Input: part model. Units: mm. Frame: model coordinates. A direction names the side the tool comes from. Give positions to 0.01 mm unless a question says otherwise; leave off trailing zeros. Order: outer loops, then holes, each group sorted by start corner. A loop starts at its lowest first (then second) coordinate and runs counter-clockwise, first axis right, second up. Notation, with made-up numbers: (70, -30.75) - (110, -30.75) arc R23 cw to (110, 1.25) - close; hole circle Ø7 at (85.5, 74). An arc over 180 degrees is marked (long way). Answer in a Markdown table with one row per item. Add a question column.
1. Ray query, line 1 (Y direction, x = -13, z = -17); line 2 (X direction, y = 4.25, z = -113); line 3 (Z direction, x = -24, y = 4.5). Return the intervals inside material, ascending. Write a range as [from, to].
2. Contact query for flat-ended pins moving along their axis: pin 1 (10 mm diameter, centred on x = 4.5, y = 7.5, fed in from -Z); pin 2 (3.5 mm diameter, centred on y = 3, z = -133.5, fed in from +X); pin 3 (13.5 mm diameter, centred on x = -2, z = -101.5, fed in from +Y); pin 4 (2 mm diameter, centred on x = -6, y = 4.5, fed in from +Z). Output: stop coordinate, or through.
3. Section query B-B on y = 15. Return loops of the section in (x, z).
4. Section query A-A on z = -97.5. Return loops of the section in (x, y).
5. Access query for faces 1 (the face through (-7.412, 12.409, -194.498)), 2 (the face through (-23.074, 0.285, 5.322)). Directions: +Z, -Z, +X, -X, +Y, -Y. A direction counts if a zero-diameter tool reaches every point of the face in a straight line with its end or side. Return the directions, or none.
```python
from build123d import *

# Parameters (mm, degrees)
SKETCH1_W           = 15
SKETCH1_H           = 200
SKETCH1_W_2         = 47.5
SKETCH1_H_2         = 10
BOSS_EXTRUDE1_DEPTH = 5
SKETCH4_R           = 2
BOSS_EXTRUDE3_DEPTH = 15
FILLET5_R           = 1
FILLET6_R           = 1


with BuildPart() as part:
    # Sketch1 → Boss-Extrude1 (new body)
    with BuildSketch(Plane(origin=(0, 0, 0), x_dir=(1, 0, 0), z_dir=(0, 1, 0))):
        Polygon((-31.25, -10), (16.25, -10), (0, 0), (-15, 0), align=None)
        with Locations((-7.5, 100)):
            Rectangle(SKETCH1_W, SKETCH1_H)
        with Locations((-7.5, -15)):
            Rectangle(SKETCH1_W_2, SKETCH1_H_2)
    extrude(amount=BOSS_EXTRUDE1_DEPTH)

    # Sketch4 → Boss-Extrude3 (add)
    with BuildSketch(Plane(origin=(0, 5, 0), x_dir=(1, 0, 0), z_dir=(0, 1, 0))):
        with Locations(Location((-7.5, 192.5, 0), (0, 0, 270))):
            Circle(SKETCH4_R)
    extrude(amount=BOSS_EXTRUDE3_DEPTH)

    # Fillet5
    fillet5_edges = [part.edges().sort_by_distance(p)[0] for p in [
        (-31.25, 5, 15),
        (-7.5, 0, -200),
        (0, 0, -100),
        (8.125, 0, 5),
        (16.25, 0, 15),
        (-7.5, 0, 20),
        (-31.25, 0, 15),
        (-23.125, 0, 5),
        (-7.5, 5, 20),
        (-15, 2.5, 0),
        (-15, 2.5, -200),
        (0, 2.5, -200),
        (0, 2.5, 0),
        (16.25, 2.5, 10),
        (-31.25, 2.5, 10),
        (16.25, 5, 15),
        (8.125, 5, 5),
        (-7.5, 5, -194.5),
        (-7.5, 20, -194.5),
        (0, 5, -100),
        (-7.5, 5, -200),
        (-15, 5, -100),
        (-23.125, 5, 5),
        (-15, 0, -100),
    ]]
    fillet(fillet5_edges, radius=FILLET5_R)

    # Fillet6
    # the kernel refuses this fillet: 1 mm, written as the material it takes off along each edge
    with BuildSketch(Plane(origin=(15.25, 4, 19), x_dir=(1, 0, 0), z_dir=(0, 0, 1))) as fillet6_piece_1_section:
        Polygon((0, 0), (FILLET6_R, 0), (FILLET6_R, FILLET6_R), (0, FILLET6_R), align=None)
    fillet6_piece_1 = extrude(amount=FILLET6_R, mode=Mode.PRIVATE)
    fillet6_piece_1 = fillet6_piece_1 - Plane(origin=(15.25, 4, 19), x_dir=(-0.7071067811865475, -0.7071067811865475, 0), z_dir=(0, 0, 1)) * Sphere(FILLET6_R, mode=Mode.PRIVATE)
    add(fillet6_piece_1, mode=Mode.SUBTRACT)
    with BuildSketch(Plane(origin=(15.25, 1, 19), x_dir=(1, 0, 0), z_dir=(0, 0, 1))) as fillet6_piece_2_section:
        Polygon((0, 0), (FILLET6_R, 0), (FILLET6_R, -FILLET6_R), (0, -FILLET6_R), align=None)
    fillet6_piece_2 = extrude(amount=FILLET6_R, mode=Mode.PRIVATE)
    fillet6_piece_2 = fillet6_piece_2 - Plane(origin=(15.25, 1, 19), x_dir=(-0.7071067811865475, 0.7071067811865475, 0), z_dir=(0, 0, 1)) * Sphere(FILLET6_R, mode=Mode.PRIVATE)
    add(fillet6_piece_2, mode=Mode.SUBTRACT)
    with BuildSketch(Plane(origin=(-30.25, 4, 19), x_dir=(0, 0, 1), z_dir=(-1, 0, 0))) as fillet6_piece_3_section:
        Polygon((0, 0), (FILLET6_R, 0), (FILLET6_R, FILLET6_R), (0, FILLET6_R), align=None)
    fillet6_piece_3 = extrude(amount=FILLET6_R, mode=Mode.PRIVATE)
    fillet6_piece_3 = fillet6_piece_3 - Plane(origin=(-30.25, 4, 19), x_dir=(0, -0.7071067811865475, -0.7071067811865475), z_dir=(-1, 0, 0)) * Sphere(FILLET6_R, mode=Mode.PRIVATE)
    add(fillet6_piece_3, mode=Mode.SUBTRACT)
    with BuildSketch(Plane(origin=(-30.25, 1, 19), x_dir=(0, 0, 1), z_dir=(-1, 0, 0))) as fillet6_piece_4_section:
        Polygon((0, 0), (FILLET6_R, 0), (FILLET6_R, -FILLET6_R), (0, -FILLET6_R), align=None)
    fillet6_piece_4 = extrude(amount=FILLET6_R, mode=Mode.PRIVATE)
    fillet6_piece_4 = fillet6_piece_4 - Plane(origin=(-30.25, 1, 19), x_dir=(0, 0.7071067811865475, -0.7071067811865475), z_dir=(-1, 0, 0)) * Sphere(FILLET6_R, mode=Mode.PRIVATE)
    add(fillet6_piece_4, mode=Mode.SUBTRACT)
    with BuildSketch(Plane(origin=(-31.25, 1, 20), x_dir=(0, 0, -1), z_dir=(0, 1, 0)), Plane(origin=(16.25, 1, 20), x_dir=(-1, 0, 0), z_dir=(0, 1, 0))) as fillet6_piece_5:
        with BuildLine():
            CenterArc((FILLET6_R, -FILLET6_R), FILLET6_R, 90, 90)
            Line((0, -FILLET6_R), (0, 0))
            Line((0, 0), (FILLET6_R, 0))
        make_face()
    extrude(amount=3, mode=Mode.SUBTRACT)


solid = part.part
```
Answer:
| question | item | result |
|---|---|---|
| 1 | line 1 | y = [0, 5] |
| 1 | line 2 | x = [-14.97, -0.03] |
| 1 | line 3 | z = [5.7, 19.87] |
| 2 | pin 1 | stops at z = 0.45 |
| 2 | pin 2 | stops at x = 0 |
| 2 | pin 3 | stops at y = 5 |
| 2 | pin 4 | stops at z = 20 |
| 3 | outline | circle Ø4 at (-7.5, -192.5) |
| 4 | outline | (-15, 1) arc R1 ccw to (-14, 0) - (-1, 0) arc R1 ccw to (0, 1) - (0, 4) arc R1 ccw to (-1, 5) - (-14, 5) arc R1 ccw to (-15, 4) - close |
| 5 | face 1 | +Y |
| 5 | face 2 | -Z, -X, -Y |
